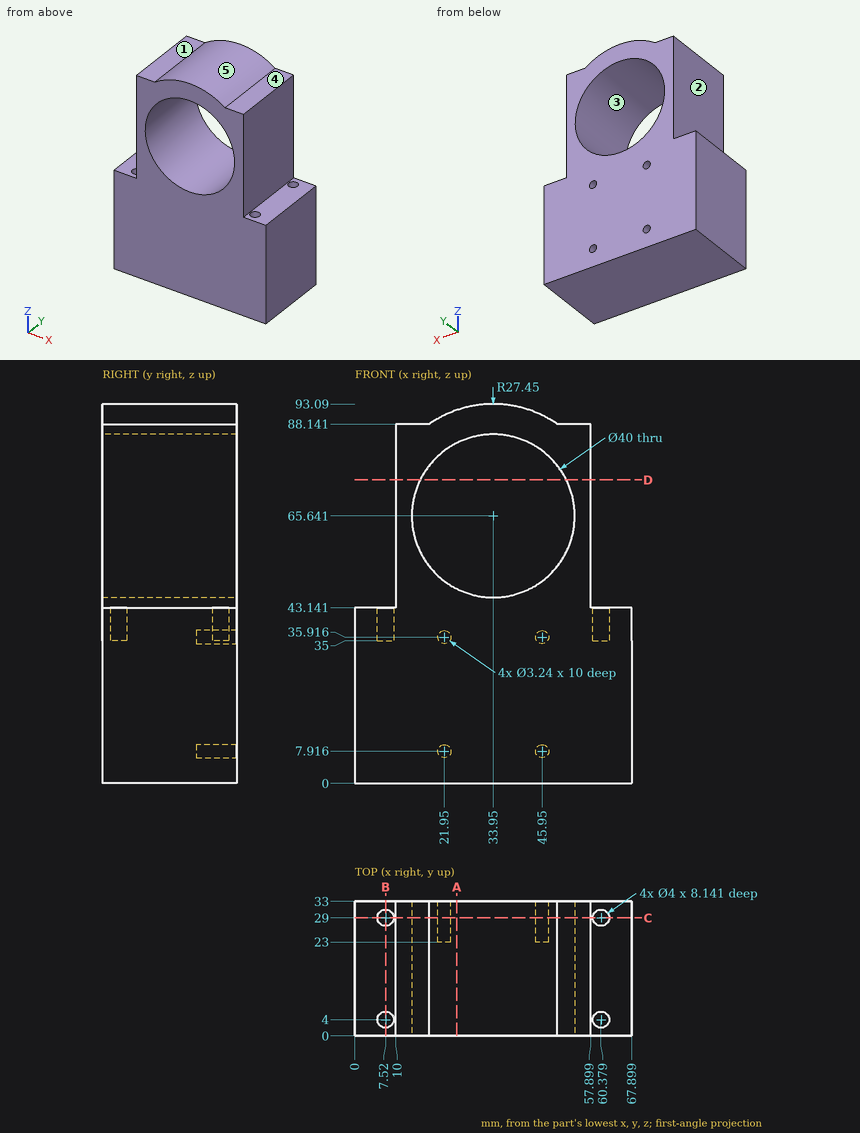
Can you work these out from the drawing? Everything is in mm from the part's minimum corner. A direction names the side the tool comes from. Round coordinates to 2 decimals unless told otherwise and drop trailing zeros. Order: outer loops, then holes, each group sorted by start corner. A loop starts at its lowest first (then second) coordinate and runs counter-clockwise, first axis right, second up. Notation, with made-up numbers: M -37,-29 L -26,-29 A6 ccw -26,-21 Z; hole C -30,-36 d8. An arc over 180 degrees is marked long. One line per question, with ' | ' between items.
1) I want a section at C-C, the plane y = 29. State how many separate pieces and enclosed holes the cut face has, then the cut area to 3 significant figures.
Working result:
separate pieces: 1 | enclosed holes: 5 | area: 3,840 mm²
2) I want a section at D-D, the plane z = 74.5. Write out the boundary of the cut face in (x, y), then the cut area to 3 significant figures.
Working result:
outline: M 10,0 L 16.02,0 L 16.02,33 L 10,33 Z; M 51.88,0 L 57.9,0 L 57.9,33 L 51.88,33 Z | area: 397 mm²
3) For pin 1 Ø9 at (x, y) = (16, 20) entering from +Z; pin 2 Ø2.5 at (x, y) = (52, 23) entering from +Z; pin 3 Ø3 at (x, y) = (6.5, 3) entering from +Z, each with a flat end and sliding along its axis, tell me the tip position at first contact or that it passes through.
Working result:
pin 1: z = 89.57 | pin 2: z = 88.14 | pin 3: z = 43.14
4) I want a section at B-B, the plane x = 7.52. Write out the boundary of the cut face in (y, z), then the cut area to 3 significant figures.
Working result:
outline: M 0,0 L 33,0 L 33,43.14 L 31,43.14 L 31,35 L 27,35 L 27,43.14 L 6,43.14 L 6,35 L 2,35 L 2,43.14 L 0,43.14 Z | area: 1,360 mm²
5) If we mould it in two halves opening along Z, with no side actions, what happens to the marked faces 1, 2 and 3? For each: +Z half, -Z half, draft (parallel to the pull), parting line (faces both ways), or undercut.
Working result:
face 1: +Z half | face 2: draft | face 3: undercut
6) I want a section at A-A, the plane x = 25. Write out the boundary of the cut face in (y, z) (1 decimal), then the cut area to 3 significant figures.
Working result:
outline: M 0,0 L 33,0 L 33,47.8 L 0,47.8 Z; M 0,83.5 L 33,83.5 L 33,91.6 L 0,91.6 Z | area: 1,840 mm²
7) For the marked faces 4 and 5, which set-ups out of +Z, -Z, +X, -X, +Y, -Y let a thin tool reach every point of the face, with its end or its side?
Working result:
face 4: +Z, +X, +Y, -Y | face 5: +Z, +Y, -Y
8) I need wall thicknesses on line 1 along Y through (x, z) = (7.52, 37.25); line 2 along Z through (x, y) = (33.5, 15) (1 decimal); line 3 along X through (y, z) = (24.5, 61) (1 decimal). Which ranges of each line are inside material? Lowest first, please.
Working result:
line 1: 0 to 2, 6 to 27, 31 to 33 | line 2: 0 to 45.6, 85.6 to 93.1 | line 3: 10 to 14.5, 53.4 to 57.9
